Build history of the part. All positions in model axes, mm. Face numbers are marked on the shaded views. A direction names the side the tool comes from. Coordinates: 2 decimals unless noted, no trailing zeros. Loops run counter-clockwise (first coordinate to the right, second up) from the corner with the lowest first, then second, coordinate; pieces in that order, holes last.
Item 1: Flat gauge pins, fed straight in: pin 1 (12 mm diameter, centred on x = 0.5, z = 43.5, fed in from +Y); pin 2 (22.5 mm diameter, centred on x = -19.19, y = -13.65, fed in from -Z) (1 decimal); pin 3 (18 mm diameter, centred on y = 38.5, z = 32, fed in from -X); pin 4 (1.5 mm diameter, centred on x = 6.5, y = 15, fed in from +Z). Where does each tip first touch, or does it go through?
Item 2: Cut at C-C (x = -9). List the corners of the cut face in (y, z).
Item 3: 3-axis set-ups, long thin cutter, end or side, ignore diameter. For the marked faces 1, 2 and 3: which of +Z, -Z, +X, -X, +Y, -Y reach the whole face in a straight line?
Item 4: Drill centre lines: line 1 along Y through (x, z) = (-19, 23); line 2 along Y through (x, z) = (-34, 58); line 3 along X through (y, z) = (34, 12). Where is each one in solid material? Low to high.
Item 5: Cut at A-A (z = 56). List the corners of the cut face in (x, y).
Item 6: Cut at B-B (y = -8.5). List the corners of the cut face in (x, z), and give its area (3 significant figures).
Item 7: Cut at D-D (y = -24). List the corners of the cut face in (x, z).
Item 8: Mould opens along X. For the marked faces 4, 5, 6 and 7 say: released by +X, released by -X, zero draft, split by the parting line, or undercut.
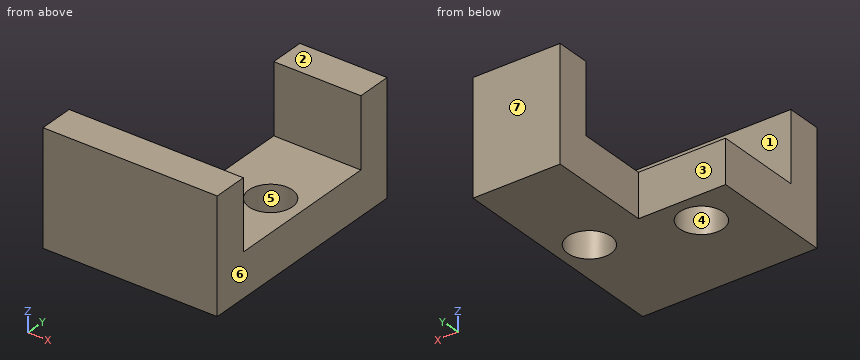
from build123d import *

# Parameters (mm, degrees)
F0_R     = 12.5
F1_DEPTH = 25
F2_W     = 100
F2_H     = 20
F2_W_2   = 50
F3_DEPTH = 40


with BuildPart() as f1:
    # F0 (on Top) → F1 (new body)
    with BuildSketch(Plane.XY):
        Polygon((-46.945058, -65.1706), (53.054942, -65.1706), (53.054942, 4.8294), (53.054942, 64.8294), (3.054942, 64.8294), (3.054942, 4.8294), (-46.945058, 4.8294), align=None)
        with Locations((-19.190943, -13.653258)):
            Circle(F0_R, mode=Mode.SUBTRACT)
        with Locations((34.849223, 0)):
            Circle(F0_R, mode=Mode.SUBTRACT)
    extrude(amount=F1_DEPTH)

    # F2 (on face) → F3 (join)
    with BuildSketch(Plane.XY.offset(25)):
        with Locations((3.054942, -55.1706)):
            Rectangle(F2_W, F2_H)
        with Locations((28.054942, 54.8294)):
            Rectangle(F2_W_2, F2_H)
    extrude(amount=F3_DEPTH)


solid = f1.part
Filled sheet:
1. pin 1: stops at y = 64.83
1. pin 2: passes through
1. pin 3: stops at x = 3.05
1. pin 4: stops at z = 25
2. outline: (-65.17, 0) - (-20.89, 0) - (-20.89, 25) - (-45.17, 25) - (-45.17, 65) - (-65.17, 65) - close; (-6.41, 0) - (4.83, 0) - (4.83, 25) - (-6.41, 25) - close
3. face 1: +Z, +X, -X
3. face 2: +Z, +X, -X, +Y, -Y
3. face 3: +Z, -Z, -X, +Y
4. line 1: y = -65.17 to -26.15, -1.15 to 4.83
4. line 2: y = -65.17 to -45.17
4. line 3: x = 3.05 to 53.05
5. outline: (-46.95, -65.17) - (53.05, -65.17) - (53.05, -45.17) - (-46.95, -45.17) - close; (3.05, 44.83) - (53.05, 44.83) - (53.05, 64.83) - (3.05, 64.83) - close
6. outline: (-46.95, 0) - (-30.58, 0) - (-30.58, 25) - (-46.95, 25) - close; (-7.8, 0) - (25.68, 0) - (25.68, 25) - (-7.8, 25) - close; (44.01, 0) - (53.05, 0) - (53.05, 25) - (44.01, 25) - close
6. area: 1,470 mm2
7. outline: (-46.95, 0) - (-26.2, 0) - (-26.2, 25) - (-46.95, 25) - close; (-12.18, 0) - (53.05, 0) - (53.05, 25) - (-12.18, 25) - close
8. face 4: undercut
8. face 5: undercut
8. face 6: released by +X
8. face 7: zero draft
